```python
from build123d import *

# Parameters (mm, degrees)
BOX006_W               = 10
BOX006_H               = 154
BOX006_DEPTH           = 4.5
BOX006_PLACEMENT_ANGLE = 307
BOX001_W               = 10
BOX001_H               = 232
BOX001_DEPTH           = 4.5
BOX_W                  = 10
BOX_H                  = 232
BOX_DEPTH              = 4.5
PAD001_DEPTH           = 4.5


with BuildPart() as front_spar001:
    # Box006 → Box006 (new body)
    with BuildSketch(Plane.XY):
        with Locations((5, 77)):
            Rectangle(BOX006_W, BOX006_H)
    extrude(amount=BOX006_DEPTH)


with BuildPart() as front_spar001_1:
    # Box006 placement: moved
    add(front_spar001.part.moved(Location((34.287817, 50.032507, -2.4))).rotate(Axis((34.287817, 50.032507, -2.4), (0, 0, 1)), BOX006_PLACEMENT_ANGLE))


with BuildPart() as cube001:
    # Box001 → Box001 (new body)
    with BuildSketch(Plane(origin=(164.7, -92.4, 2.5), x_dir=(1, 0, 0), z_dir=(0, 0, 1))):
        with Locations((5, 116)):
            Rectangle(BOX001_W, BOX001_H)
    extrude(amount=BOX001_DEPTH)


with BuildPart() as cube:
    # Box → Box (new body)
    with BuildSketch(Plane(origin=(190, -89.9, 2.5), x_dir=(1, 0, 0), z_dir=(0, 0, 1))):
        with Locations((5, 116)):
            Rectangle(BOX_W, BOX_H)
    extrude(amount=BOX_DEPTH)


with BuildPart() as cut035:
    # Sketch001 → Pad001 (new body)
    with BuildSketch(Plane.XZ):
        Polygon((-112.766838, 5.66261), (-112.766838, -1.625728), (3.473136, -43.933619), (3.473136, 47.970501), align=None)
    extrude(amount=PAD001_DEPTH)


with BuildPart() as cut035_1:
    # Body001 placement: moved
    add(cut035.part.moved(Location((250, 135, -4))))

    # Cut011: cut Cube
    add(cube.part, mode=Mode.SUBTRACT)

    # Cut023: cut Cube001
    add(cube001.part, mode=Mode.SUBTRACT)

    # Cut035: cut front spar001
    add(front_spar001_1.part, mode=Mode.SUBTRACT)


solid = cut035_1.part
```
Build history of the part. All positions in model axes, mm. A direction names the side the tool comes from. Round coordinates to 2 decimals unless told otherwise and drop trailing zeros. Write each loop counter-clockwise with the first axis right and the second up, starting at its lowest first coordinate (ties: lowest second). Pieces come first, ordered by that corner, then holes. Notation, with made-up numbers: (-17, -16.75) - (-10, -16.75) arc R22 ccw to (-10, -9.75) - close; hole circle Ø7 at (61.25, 78). An arc over 180 degrees is marked (long way). Write each question's results on one line, items separated by ' | '. Start each with the question number.
Item 1: Wall check: L1, parallel to Z at x = 168.5, y = 134.25; L2, parallel to Z at x = 244, y = 131.05; L3, parallel to Z at x = 181, y = 134.05. Give the ranges that are in metal, low to high. Write a range as [from, to].
Item 2: Mould opens along Z. For faces 6 (the face through (195, 133, 7)), 7 (the face through (196.167, 132.782, 23.113)), 8 (the face through (220, 130.5, -1)) say: pulls with the +Z half, pulls with the -Z half, needs draft (parallel to the pull), parting line crosses it, or undercut.
Item 3: Drop flat-ended pins along their axis: P1, Ø1, axis at x = 195, y = 134, coming from the +Z side; P2, Ø2, axis at x = 155.5, y = 132.5, coming from the -Z side; P3, Ø2, axis at x = 167.5, y = 134, coming from the +Z side. Give the stop position or say it passes through.
Item 4: Which spindle directions (+Z, -Z, +X, -X, +Y, -Y) get a long thin tool onto all of the face, cutting with end or side? Do faces 1 (the face through (253.473, 133, -3)), 2 (the face through (170, 133, 2.5)), 3 (the face through (194.539, 132.782, -26.484)), 4 (the face through (144.02, 132.72, -0.18)), 5 (the face through (152, 133, -2.4)). Say none if no direction does.
Item 5: Saw through at A-A (z = -1). Write the cut outline in (x, y).
Item 6: Saw through at B-B (x = 151). Write the cut outline in (y, z).
Item 7: Saw through at C-C (y = 132.3). Write the cut outline in (x, z), and give its area (3 significant figures).
Item 8: Saw through at D-D (z = -13). Write the cut outline in (x, y).
Results are:
1) L1: z = [-17.01, 2.5], [7, 13.04] | L2: z = [-44.49, 40.52] | L3: z = [-21.56, 17.59]
2) face 6: undercut | face 7: pulls with the +Z half | face 8: needs draft
3) P1: stops at z = 22.87 | P2: stops at z = -12.64 | P3: stops at z = 13.04
4) face 1: +Z, -Z, +X, +Y, -Y | face 2: +Y, -Y | face 3: -Z, -X, +Y, -Y | face 4: -Y | face 5: none
5) outline: (137.23, 130.5) - (141.07, 130.5) - (147.04, 135) - (137.23, 135) - close; (157.69, 130.5) - (253.47, 130.5) - (253.47, 135) - (163.09, 135) - (163.3, 134.73) - close
6) outline: (130.5, -10.64) - (135, -10.64) - (135, -2.4) - (130.5, -2.4) - close; (130.5, 2.1) - (135, 2.1) - (135, 6.67) - (130.5, 6.67) - close
7) outline: (137.23, -5.63) - (253.47, -47.93) - (253.47, 43.97) - (137.23, 1.66) - close; hole (143.46, -2.4) - (160.08, -2.4) - (160.08, 2.1) - (143.46, 2.1) - close; hole (164.7, 2.5) - (174.7, 2.5) - (174.7, 7) - (164.7, 7) - close; hole (190, 2.5) - (200, 2.5) - (200, 7) - (190, 7) - close | area: 5,600 mm²
8) outline: (157.49, 130.5) - (253.47, 130.5) - (253.47, 135) - (157.49, 135) - close
